Source: three-view drawing plus pictorial views. Frame: mm from the lowest corner of the part. Give positions to 0.01 mm unless a question says otherwise; leave off trailing zeros. Loops run counter-clockwise (first coordinate to the right, second up) from the corner with the lowest first, then second, coordinate; pieces in that order, holes last. Notation, with made-up numbers: (63, 48.5) - (67, 48.5) arc R33 cw to (67, 78.5) - close; hole circle Ø3 at (49, 46.25). An arc over 180 degrees is marked (long way). Put each result on its own line as item: value.
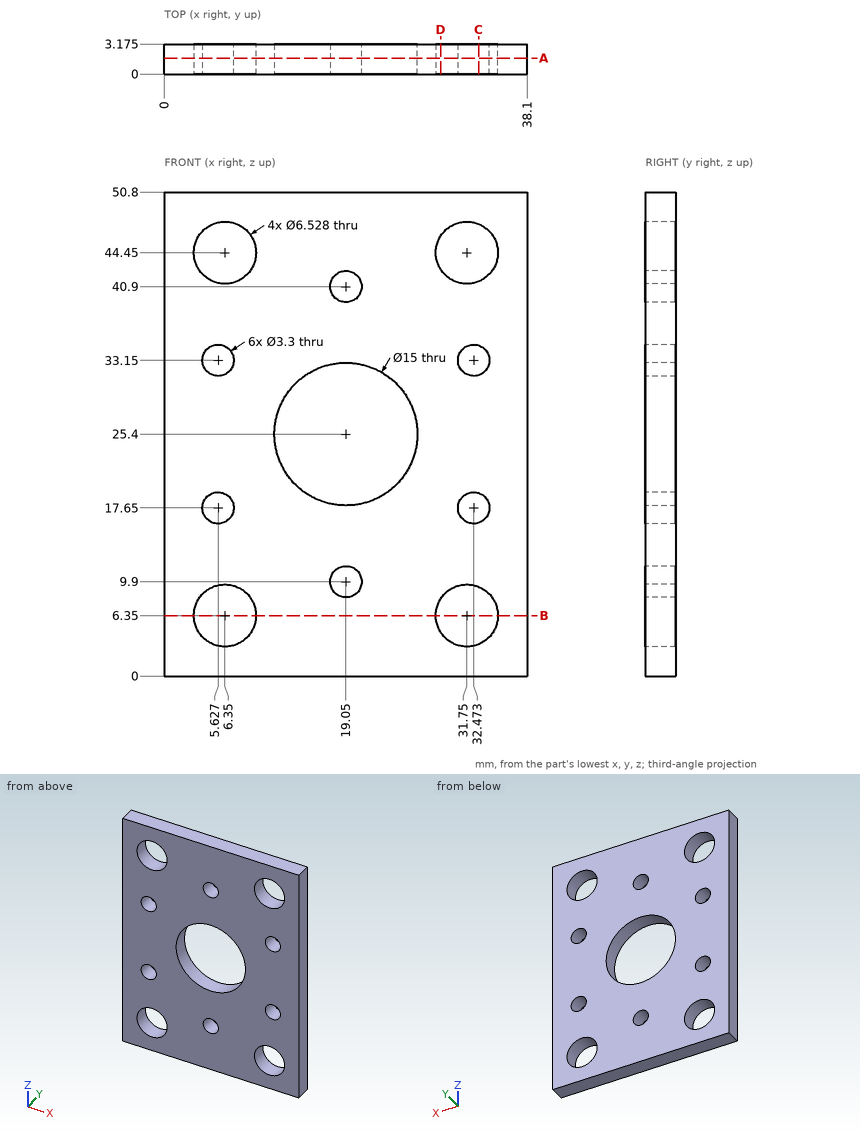
1) Section query C-C, the plane x = 33. Output: boundary loops of the cut face in (y, z) (1 decimal), plus the area to 3 significant figures.
Check result:
outline: (0, 0) - (3.2, 0) - (3.2, 3.3) - (0, 3.3) - close; (0, 9.4) - (3.2, 9.4) - (3.2, 16.1) - (0, 16.1) - close; (0, 19.2) - (3.2, 19.2) - (3.2, 31.6) - (0, 31.6) - close; (0, 34.7) - (3.2, 34.7) - (3.2, 41.4) - (0, 41.4) - close; (0, 47.5) - (3.2, 47.5) - (3.2, 50.8) - (0, 50.8) - close
area: 103 mm²
2) Section query D-D, the plane x = 29. Output: boundary loops of the cut face in (y, z) (1 decimal).
Check result:
outline: (0, 0) - (3.2, 0) - (3.2, 4.6) - (0, 4.6) - close; (0, 8.1) - (3.2, 8.1) - (3.2, 42.7) - (0, 42.7) - close; (0, 46.2) - (3.2, 46.2) - (3.2, 50.8) - (0, 50.8) - close
3) Material intervals for line 1 along X through (y, z) = (2.45, 6.35); line 2 along Z through (x, y) = (19.05, 1.35); line 3 along Z through (x, y) = (31.75, 2.5) (1 decimal), sorted ascending. Write a range as [from, to].
Check result:
line 1: [0, 3.09], [9.61, 28.49], [35.01, 38.1]
line 2: [0, 8.25], [11.55, 17.9], [32.9, 39.25], [42.55, 50.8]
line 3: [0, 3.1], [9.6, 16.2], [19.1, 31.7], [34.6, 41.2], [47.7, 50.8]
4) Pin query (flat end, axial travel): P1, Ø4.5, axis at x = 32.47, z = 33.15, coming from the +Y side (3 decimals). Return the tip coordinate at first contact, or that it passes through.
Check result:
P1: y = 3.175
5) Section query B-B, the plane z = 6.35. Output: boundary loops of the cut face in (x, y) (1 decimal).
Check result:
outline: (0, 0) - (3.1, 0) - (3.1, 3.2) - (0, 3.2) - close; (9.6, 0) - (28.5, 0) - (28.5, 3.2) - (9.6, 3.2) - close; (35, 0) - (38.1, 0) - (38.1, 3.2) - (35, 3.2) - close
6) Section query A-A, the plane y = 1.7. State how many separate pieces and enclosed holes the cut face has, plus the area to 3 significant figures.
Check result:
separate pieces: 1
enclosed holes: 11
area: 1,570 mm²
